Check sheet for the modelled part. Datum: model origin and axes. Units: mm. Face numbers are marked on the shaded views. A direction names the side the tool comes from. Coordinates: 2 decimals unless noted, no trailing zeros. Write each loop counter-clockwise with the first axis right and the second up, starting at its lowest first coordinate (ties: lowest second). Pieces come first, ordered by that corner, then holes. Notation, with made-up numbers: M 89.25,71.5 L 134.25,71.5 A11 ccw 134.25,84.5 Z; hole C -14.5,34 d4. An arc over 180 degrees is marked long. Answer as CSV lines item,"result".
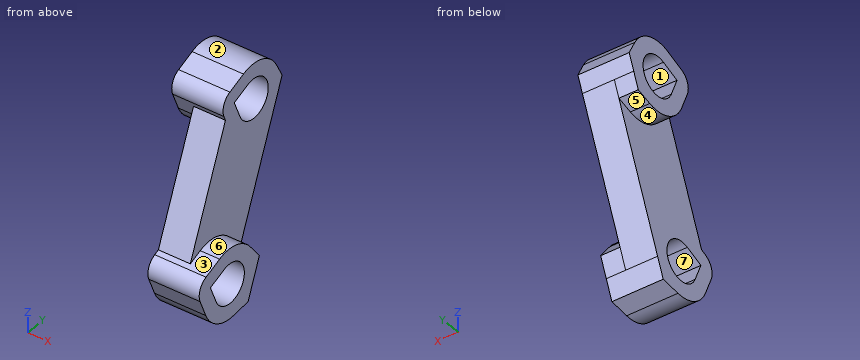
Autodesk Inventor part; units mm, degrees
ref_plane "YZ Plane" through (0, 0, 0) normal (1, 0, 0) x (0, 1, 0)
ref_plane "XY Plane" through (0, 0, 0) normal (0, 0, 1) x (1, 0, 0)
sketch "スケッチ1" plane through (0, 0, 0) normal (1, 0, 0) x (0, 1, 0)
  arc A0 (-2.7792, 1.1297) -> (2.7792, -1.1297) centre (0, 0) ccw
  circle A1 centre (5, 12.3) radius 1.7
  arc A2 (7.7792, 11.1703) -> (2.2208, 13.4297) centre (5, 12.3) ccw
  circle A3 centre (0, 0) radius 1.7
  line L0 (2.2208, 13.4297) -> (-2.7792, 1.1297)
  line L1 (7.7792, 11.1703) -> (2.7792, -1.1297)
  dimension "d1" = 3.4
  dimension "d2" = 6
  dimension "d3" = 3.4
  dimension "d4" = 5
  dimension "d5" = 12.3
  dimension "d8" = 3
extrude "押し出し1" add sketch "スケッチ1" against normal blind 6.2
sketch "スケッチ2" plane through (0, 0, 0) normal (1, 0, 0) x (0, 0, -1)
  circle A0 centre (0, 0) radius 1.7
  circle A1 centre (-12.3, 5) radius 1.7
  line L0 (-1.1297, -2.7792) -> (-13.4297, 2.2208)
  arc A2 (-1.1297, -2.7792) -> (1.1297, 2.7792) centre (0, 0) ccw
  line L1 (-11.1703, 7.7792) -> (1.1297, 2.7792)
  arc A3 (-11.1703, 7.7792) -> (-13.4297, 2.2208) centre (-12.3, 5) ccw
  circle A4 centre (0, 0) radius 3
  line L2 (-1.1297, -2.7792) -> (1.1297, 2.7792)
  dimension "d11" = 6
extrude "押し出し2" cut sketch "スケッチ2" against normal blind 1.7 contours A4 L0 A3 L1
sketch "スケッチ3" plane through (-6.2, 0, 0) normal (-1, 0, 0) x (0, 0, 1)
  circle A0 centre (0, 0) radius 1.7
  circle A1 centre (12.3, 5) radius 1.7
  line L0 (1.1297, -2.7792) -> (13.4297, 2.2208)
  arc A2 (13.4297, 2.2208) -> (11.1703, 7.7792) centre (12.3, 5) ccw
  line L1 (11.1703, 7.7792) -> (-1.1297, 2.7792)
  arc A3 (-1.1297, 2.7792) -> (1.1297, -2.7792) centre (0, 0) ccw
  circle A4 centre (12.3, 5) radius 3
  line L2 (11.1703, 7.7792) -> (13.4297, 2.2208)
  line L3 (1.1297, -2.7792) -> (13.4297, 2.2208)
  dimension "d14" = 6
extrude "押し出し3" cut sketch "スケッチ3" against normal blind 1.7 contours A4 L0 A3 L1
sketch "スケッチ4" plane through (-1.7, 0, 0) normal (1, 0, 0) x (0, 0, -1)
  arc A0 (1.1297, 2.7792) -> (-1.1297, -2.7792) centre (0, 0) ccw
  line L0 (-11.1703, 7.7792) -> (1.1297, 2.7792)
  arc A1 (-11.1703, 7.7792) -> (-13.4297, 2.2208) centre (-12.3, 5) ccw
  line L1 (-1.1297, -2.7792) -> (-13.4297, 2.2208)
  circle A2 centre (-12.3, 5) radius 1.7
  line L2 (-13.4297, 2.2208) -> (-13.8977, 1.0697)
  line L3 (-13.8977, 1.0697) -> (-15.064, 3.8337)
  arc A3 (-11.1703, 7.7792) -> (-13.4297, 2.2208) centre (-12.3, 5) ccw
  dimension "d17" = 45
extrude "押し出し4" add sketch "スケッチ4" against normal up to surface (4.5 mm away) contours L2 L3 A1
mirror "ミラー1" about plane through (-1.7, 2.2208, 13.4297) normal (0, -0.3765791, -0.9263845) of "押し出し4"
sketch "スケッチ5" plane through (-1.7, 0, 0) normal (1, 0, 0) x (0, 0, -1)
  line L0 (-1.1297, -2.7792) -> (-12.2786, 1.7529)
  arc A0 (1.1297, 2.7792) -> (-1.1297, -2.7792) centre (0, 0) ccw
  line L1 (-11.1703, 7.7792) -> (1.1297, 2.7792)
  arc A1 (-11.1703, 7.7792) -> (-15.064, 3.8337) centre (-12.3, 5) ccw
  line L2 (-15.064, 3.8337) -> (-13.8977, 1.0697)
  line L3 (-12.2786, 1.7529) -> (-13.8977, 1.0697)
  circle A2 centre (-12.3, 5) radius 1.7
  line L4 (-12.9402, 3.4251) -> (-13.2054, 2.7728)
  line L5 (-13.2054, 2.7728) -> (-13.8663, 4.3391)
  circle A3 centre (-12.3, 5) radius 1.7
  arc A4 (-13.8663, 4.3391) -> (-12.9402, 3.4251) centre (-12.3, 5) ccw
  dimension "d20" = 45
extrude "押し出し5" cut sketch "スケッチ5" against normal blind 10 contours A2 L4 L5
mirror "ミラー2" about plane through (-1.7, 3.4251, 12.9402) normal (0, 0.3765791, 0.9263845) of "押し出し5"
fillet "フィレット1" radius 1.3 1 edges at (-3.95, 1.0697, 13.8977)
sketch "スケッチ6" plane through (-4.5, 0, 0) normal (-1, 0, 0) x (0, 0, 1)
  circle A0 centre (0, 0) radius 1.7
  line L0 (12.2786, 1.7529) -> (11.1337, 2.236)
  arc A1 (11.1703, 7.7792) -> (11.1337, 2.236) centre (12.3, 5) ccw
  line L1 (-1.1297, 2.7792) -> (11.1703, 7.7792)
  arc A2 (-1.1297, 2.7792) -> (1.1297, -2.7792) centre (0, 0) ccw
  line L2 (12.2786, 1.7529) -> (1.1297, -2.7792)
  line L3 (1.1297, -2.7792) -> (1.5977, -3.9303)
  line L4 (1.5977, -3.9303) -> (-1.1663, -2.764)
  dimension "d24" = 45
extrude "押し出し6" add sketch "スケッチ6" against normal up to surface (4.5 mm away) contours L3 L4 A2
mirror "ミラー3" about plane through (-4.5, -2.7792, 1.1297) normal (0, 0.3765791, 0.9263845) of "押し出し6"
sketch "スケッチ7" plane through (-4.5, 0, 0) normal (-1, 0, 0) x (0, 0, 1)
  circle A0 centre (0, 0) radius 1.7
  line L0 (0.6402, -1.5749) -> (0.9054, -2.2272)
  line L1 (0.9054, -2.2272) -> (-0.6609, -1.5663)
  line L2 (-1.1297, 2.7792) -> (11.1703, 7.7792)
  dimension "d29" = 45
extrude "押し出し7" cut sketch "スケッチ7" against normal blind 10 contours A0 L0 L1
mirror "ミラー4" about plane through (-4.5, -1.5749, 0.6402) normal (0, -0.3765791, -0.9263845) of "押し出し7"
fillet "フィレット2" radius 1.3 1 edges at (-2.25, -3.9303, 1.5977)
sketch "スケッチ8" plane through (-4.5, 0, 0) normal (-1, 0, 0) x (0, 0, 1)
  line L0 (-1.1297, 2.7792) -> (11.1703, 7.7792)
  arc A0 (-1.1297, 2.7792) -> (-1.1663, -2.764) centre (0, 0) ccw
  line L1 (-1.1297, 2.7792) -> (-2.7291, 2.129)
  line L2 (-2.7291, 2.129) -> (-2.9705, 0.4196)
extrude "押し出し8" add sketch "スケッチ8" against normal up to surface (4.5 mm away)
ref_plane "作業平面1" through (0, 2.7792, -1.1297) normal (0, -0.3765791, -0.9263845) x (-1, 0, 0)
mirror "ミラー5" about plane through (0, 2.7792, -1.1297) normal (0, -0.3765791, -0.9263845) of "押し出し8"
sketch "スケッチ9" plane through (-6.2, 0, 0) normal (-1, 0, 0) x (0, 0, 1)
  arc A0 (12.7, 1.5751) -> (14.4031, 2.2674) centre (13.2054, 2.7728) ccw
  line L0 (14.4031, 2.2674) -> (15.064, 3.8337)
  arc A1 (15.064, 3.8337) -> (11.1337, 2.236) centre (12.3, 5) ccw
  line L1 (12.7, 1.5751) -> (11.1337, 2.236)
  line L2 (13.2054, 2.7728) -> (11.6391, 3.4337)
  arc A2 (13.8663, 4.3391) -> (11.6391, 3.4337) centre (12.3, 5) ccw
  line L3 (13.8663, 4.3391) -> (13.2054, 2.7728)
  line L4 (-2.7291, 2.129) -> (11.1703, 7.7792)
  line L5 (11.1703, 7.7792) -> (12.4648, 8.3054)
  line L6 (12.4648, 8.3054) -> (13.7006, 7.653)
  point P0 (0, 0)
extrude "押し出し9" add sketch "スケッチ9" against normal up to surface (4.5 mm away) contours L5 L6 A1
ref_plane "作業平面2" through (0, 7.7792, 11.1703) normal (0, -0.3765791, -0.9263845) x (-1, 0, 0)
mirror "ミラー6" about plane through (0, 7.7792, 11.1703) normal (0, -0.3765791, -0.9263845) of "押し出し9"
ref_plane "作業平面3" through (0, 7.7792, 11.1703) normal (0, -0.3765791, -0.9263845) x (-1, 0, 0)
properties part number "HbRing-LittleCouplerLink01" material "ナイロン 6/6"
1) Section check B-B, the plane y = 5.25. Record the boundary of the cut face in (x, z), plus the area to 3 significant figures.
Answer key:
outline,"M -6.2,9.31 L -4.5,9.31 L -4.5,4.95 L -1.7,4.95 L -1.7,10.62 L -6.2,10.62 Z; M -6.2,13.98 L -1.7,13.98 L -1.7,15.29 L -6.2,15.29 Z"
area,"24.0 mm2"
2) Section check C-C, the plane x = -5.25. Record the boundary of the cut face in (y, z).
Answer key:
outline,"M 1.58,12.7 L 2.24,11.13 A3 ccw 5.92,9.45 L 7.25,9.88 L 7.78,11.17 L 8.31,12.46 L 7.65,13.7 A3 ccw 3.83,15.06 L 2.27,14.4 A1.3 ccw Z; hole M 2.77,13.21 L 3.43,11.64 A1.7 ccw long 4.34,13.87 Z"
3) Tool access check on the marked faces 4, 5, 6 and 7. Record the directions out of +Z, -Z, +X, -X, +Y, -Y that give a thin tool (end or side, any length) a straight path to the whole face; none if there is none.
Answer key:
face 4,"-Z, -X"
face 5,"-Z, -X, +Y"
face 6,"+Z, +X"
face 7,"+X, -X"
4) Section check A-A, the plane z = -0.25. Record the boundary of the cut face in (x, y).
Answer key:
outline,"M -4.5,-3.15 L 0,-3.15 L 0,-1.74 L -4.5,-1.74 Z; M -4.5,1.68 L 0,1.68 L 0,3.14 L -4.5,3.14 Z"
5) Mould release check, pull along Y, two halves, no side actions. Record for the marked faces 1, 2 and 3: pulls with the +Y half, pulls with the -Y half, needs draft (parallel to the pull), parting line crosses it, or undercut.
Answer key:
face 1,"undercut"
face 2,"parting line crosses it"
face 3,"pulls with the -Y half"
6) Thickness scan on line 1 along Z through (x, y) = (-0.9, 0); line 2 along Z through (x, y) = (-4.75, 5); line 3 along X through (y, z) = (4.25, 8.75). Record the ranges inside material, lowest first.
Answer key:
line 1,"z = -3 to -1.7, 1.7 to 3"
line 2,"z = 9.3 to 10.6, 14 to 15.3"
line 3,"x = -4.5 to -1.7"
7) Depth check by flat-ended pin: P1, Ø5, axis at y = 2, z = 11.5, coming from the +X side; P2, Ø1.5, axis at x = -2, y = 3, coming from the -Z side; P3, Ø3, axis at x = -5.5, y = 2.5, coming from the +Z side; P4, Ø2, axis at y = 5, z = 12.3, coming from the +X side. Enter the tip coordinate at first touch or a pass-through.
Answer key:
P1,"stops at x = -1.7"
P2,"stops at z = -2.43"
P3,"stops at z = 15.13"
P4,"passes through"
8) Section check D-D, the plane x = -2.5. Record the boundary of the cut face in (y, z), plus the area to 3 significant figures.
Answer key:
outline,"M -3.42,0.4 L -2.76,-1.17 A3 ccw 0.42,-2.97 L 2.13,-2.73 L 2.78,-1.13 L 7.78,11.17 L 8.31,12.46 L 7.65,13.7 A3 ccw 3.83,15.06 L 2.27,14.4 A1.3 ccw 1.58,12.7 L 1.75,12.28 L -2.31,2.28 L -2.73,2.1 A1.3 ccw Z; hole M -2.23,0.91 L -1.57,-0.66 A1.7 ccw long -0.66,1.57 Z; hole M 2.77,13.21 L 3.43,11.64 A1.7 ccw long 4.34,13.87 Z"
area,"92.0 mm2"
